Here's how the part is built. I have some questions about the finished solid (model axes, mm). Round coordinates to 2 decimals unless told otherwise and drop trailing zeros. Write each loop counter-clockwise with the first axis right and the second up, starting at its lowest first coordinate (ties: lowest second). Pieces come first, ordered by that corner, then holes. Notation, with made-up numbers: (-6.75, -7) -> (19.25, -7) arc R25 ccw to (19.25, 21) -> close; hole circle Ø5 at (69, 5.25). An arc over 180 degrees is marked (long way). Answer as CSV lines item,"result".
from build123d import *

# Parameters (mm, degrees)
SKETCH1_W           = 150
SKETCH1_H           = 70
BOSS_EXTRUDE1_DEPTH = 4
SKETCH4_R           = 12
SKETCH4_R_2         = 6
BOSS_EXTRUDE6_DEPTH = 30
LPATTERN1_COUNT     = 3
LPATTERN1_PITCH     = 60
SKETCH7_R           = 2
CUT_EXTRUDE2_DEPTH  = 30
CHAMFER3_SIZE       = 4
SKETCH8_W           = 30
SKETCH8_H           = 6
CUT_EXTRUDE3_DEPTH  = 10
SKETCH9_W           = 30
SKETCH9_H           = 5.757460858
CUT_EXTRUDE4_DEPTH  = 10


with BuildPart() as part:
    # Sketch1 → Boss-Extrude1 (new body, symmetric)
    with BuildSketch(Plane.XY):
        Rectangle(SKETCH1_W, SKETCH1_H)
    extrude(amount=BOSS_EXTRUDE1_DEPTH, both=True)

    # Sketch4 → Boss-Extrude6 (add)
    with BuildSketch(Plane(origin=(75, 0, 0), x_dir=(0, 0, -1), z_dir=(1, 0, 0))):
        with Locations((6.400440408, 40.953753189)):
            Circle(SKETCH4_R)
        with Locations((6.400440408, 40.953753189)):
            Circle(SKETCH4_R_2, mode=Mode.SUBTRACT)
    boss_extrude6 = extrude(amount=-BOSS_EXTRUDE6_DEPTH)

    # LPattern1: Boss-Extrude6 ×3
    with Locations(*[(-i * LPATTERN1_PITCH, 0, 0) for i in range(1, LPATTERN1_COUNT)]):
        add(boss_extrude6)

    # Sketch7 → Cut-Extrude2 (cut)
    with BuildSketch(Plane.XY.offset(4)):
        with Locations((-56.630501899, 15.015863732)):
            Circle(SKETCH7_R)
        with Locations((0, -21.058085924)):
            Circle(SKETCH7_R)
        with Locations((61.669656729, 15.015863732)):
            Circle(SKETCH7_R)
    extrude(amount=-CUT_EXTRUDE2_DEPTH, mode=Mode.SUBTRACT)

    # Chamfer3
    chamfer3_edges = [part.edges().sort_by_distance(p)[0] for p in [
        (-58.630501899, 15.015863732, -4),
        (-2, -21.058085924, -4),
        (59.669656729, 15.015863732, -4),
    ]]
    chamfer(chamfer3_edges, length=CHAMFER3_SIZE)

    # Sketch8 → Cut-Extrude3 (cut)
    with BuildSketch(Plane(origin=(0, 0, -4), x_dir=(-1, 0, 0), z_dir=(0, 0, -1))):
        with Locations((-30, 31.953753189)):
            Rectangle(SKETCH8_W, SKETCH8_H)
    extrude(amount=-CUT_EXTRUDE3_DEPTH, mode=Mode.SUBTRACT)

    # Sketch9 → Cut-Extrude4 (cut)
    with BuildSketch(Plane(origin=(0, 0, -4), x_dir=(-1, 0, 0), z_dir=(0, 0, -1))):
        with Locations((30, 32.07502276)):
            Rectangle(SKETCH9_W, SKETCH9_H)
    extrude(amount=-CUT_EXTRUDE4_DEPTH, mode=Mode.SUBTRACT)


solid = part.part
Item 1: Suppose I cut it at B-B, the plane z = -8.5. List the corners of the cut face in (x, y) for me.
Results found:
outline,"(-75, 29.14) -> (-45, 29.14) -> (-45, 35.33) -> (-75, 35.33) -> close; (-75, 46.57) -> (-45, 46.57) -> (-45, 52.77) -> (-75, 52.77) -> close; (-15, 29.14) -> (15, 29.14) -> (15, 35.33) -> (-15, 35.33) -> close; (-15, 46.57) -> (15, 46.57) -> (15, 52.77) -> (-15, 52.77) -> close; (45, 29.14) -> (75, 29.14) -> (75, 35.33) -> (45, 35.33) -> close; (45, 46.57) -> (75, 46.57) -> (75, 52.77) -> (45, 52.77) -> close"
Item 2: I need wall thicknesses on L1, parallel to X at y = 33, z = -2.75; L2, parallel to X at y = 16.5, z = -3.5; L3, parallel to Z at x = -42.5, y = 16.5. Which ranges of each line are inside material? Lowest first, please.
Results found:
L1,"x = -75 to -45, -15 to 15, 45 to 75"
L2,"x = -75 to -61.93, -51.33 to 56.37, 66.97 to 75"
L3,"z = -4 to 4"
Item 3: Suppose I cut it at C-C, the plane y = 37. List the corners of the cut face in (x, z) for me, then the cut area to 3 significant figures.
Results found:
outline,"(-75, -17.73) -> (-45, -17.73) -> (-45, -10.91) -> (-75, -10.91) -> close; (-75, -1.89) -> (-45, -1.89) -> (-45, 4.93) -> (-75, 4.93) -> close; (-15, -17.73) -> (15, -17.73) -> (15, -10.91) -> (-15, -10.91) -> close; (-15, -1.89) -> (15, -1.89) -> (15, 4.93) -> (-15, 4.93) -> close; (45, -17.73) -> (75, -17.73) -> (75, -10.91) -> (45, -10.91) -> close; (45, -1.89) -> (75, -1.89) -> (75, 4.93) -> (45, 4.93) -> close"
area,"1,230 mm²"
Item 4: Will these pins go through, and if not, where does the flat tip stop? pin 1 (10 mm diameter, centred on x = 47.5, z = -12.5, fed in from +Y); pin 2 (10 mm diameter, centred on y = -13, z = -13, fed in from +X); pin 3 (8 mm diameter, centred on x = 55, y = 6.5, fed in from +Z); pin 4 (14 mm diameter, centred on y = 40.95, z = -6.4, fed in from +X).
Results found:
pin 1,"stops at y = 52.9"
pin 2,"passes through"
pin 3,"stops at z = 4"
pin 4,"stops at x = 75"
Item 5: If we mould it in two halves opening along Y, with no side actions, what happens to faces 1 (the flat face through (30, 28.954, 0)), 2 (the flat face through (-1, 0, 4)), 3 (the flat face through (-30, 29.196, 0))? For each: pulls with the +Y half, pulls with the -Y half, needs draft (parallel to the pull), parting line crosses it, or undercut.
Results found:
face 1,"undercut"
face 2,"needs draft"
face 3,"undercut"
Item 6: Suppose I cut it at A-A, the plane x = 28.5. List the corners of the cut face in (y, z) for me.
Results found:
outline,"(-35, -4) -> (28.95, -4) -> (28.95, 4) -> (-35, 4) -> close; (34.95, -4) -> (35, -4) -> (35, 4) -> (34.95, 4) -> close"
Item 7: Suppose I cut it at D-D, the plane x = 0. List the corners of the cut face in (y, z) for me.
Results found:
outline,"(-35, -4) -> (-27.06, -4) -> (-23.06, 0) -> (-23.06, 4) -> (-35, 4) -> close; (-19.06, 0) -> (-15.06, -4) -> (29.2, -4) arc R12 ccw (long way) to (34.97, 4) -> (-19.06, 4) -> close; hole circle Ø12 at (40.95, -6.4)"
